Input: part model. Units: mm. Frame: model coordinates. A direction names the side the tool comes from. Give positions to 0.01 mm unless a question says otherwise; leave off trailing zeros. Loops run counter-clockwise (first coordinate to the right, second up) from the corner with the lowest first, then second, coordinate; pieces in that order, holes last. Notation, with made-up numbers: (26.5, 53) - (53.5, 53) arc R13 cw to (53.5, 72) - close; hole circle Ø11 at (-22.75, 12.25). An arc over 180 degrees is marked (long way). Answer as a JSON object with one key per item and string values.
from build123d import *

# Parameters (mm, degrees)
SKETCH1_W           = 106
SKETCH1_H           = 6
BOSS_EXTRUDE1_DEPTH = 6
SKETCH2_W           = 6
SKETCH2_H           = 20
SKETCH2_R           = 1.75
BOSS_EXTRUDE2_DEPTH = 6
FILLET1_R           = 2


with BuildPart() as part:
    # Sketch1 → Boss-Extrude1 (new body)
    with BuildSketch(Plane(origin=(0, 0, 0), x_dir=(1, 0, 0), z_dir=(0, 1, 0))):
        Rectangle(SKETCH1_W, SKETCH1_H)
    extrude(amount=BOSS_EXTRUDE1_DEPTH)

    # Sketch2 → Boss-Extrude2 (add)
    # profile 1 of 4: a face of its own
    with BuildSketch(Plane(origin=(0, 6, 0), x_dir=(1, 0, 0), z_dir=(0, 1, 0))):
        with Locations((-50, 13)):
            Rectangle(SKETCH2_W, SKETCH2_H)
        with Locations(Location((-50, 20, 0), (0, 0, 270))):
            Circle(SKETCH2_R, mode=Mode.SUBTRACT)
    # profile 2 of 4: a face of its own
    with BuildSketch(Plane(origin=(0, 6, 0), x_dir=(1, 0, 0), z_dir=(0, 1, 0))):
        with Locations((-50, -13)):
            Rectangle(SKETCH2_W, SKETCH2_H)
        with Locations(Location((-50, -20, 0), (0, 0, 90))):
            Circle(SKETCH2_R, mode=Mode.SUBTRACT)
    # profile 3 of 4: a face of its own
    with BuildSketch(Plane(origin=(0, 6, 0), x_dir=(1, 0, 0), z_dir=(0, 1, 0))):
        with Locations((50, -13)):
            Rectangle(SKETCH2_W, SKETCH2_H)
        with Locations(Location((50, -20, 0), (0, 0, 270))):
            Circle(SKETCH2_R, mode=Mode.SUBTRACT)
    # profile 4 of 4: a face of its own
    with BuildSketch(Plane(origin=(0, 6, 0), x_dir=(1, 0, 0), z_dir=(0, 1, 0))):
        with Locations((50, 13)):
            Rectangle(SKETCH2_W, SKETCH2_H)
        with Locations(Location((50, 20, 0), (0, 0, 90))):
            Circle(SKETCH2_R, mode=Mode.SUBTRACT)
    extrude(amount=-BOSS_EXTRUDE2_DEPTH)

    # Fillet1
    fillet1_edges = [part.edges().sort_by_distance(p)[0] for p in [
        (-47, 3, -3),
        (-47, 3, 3),
        (47, 3, 3),
        (47, 3, -3),
    ]]
    fillet(fillet1_edges, radius=FILLET1_R)


solid = part.part
Item 1: Cut plane B-B (x = 50). Return loops of the section in (y, z), then the cut area to 3 significant figures.
Geometry check:
{"outline": "(0, -23) - (6, -23) - (6, -21.75) - (0, -21.75) - close; (0, -18.25) - (6, -18.25) - (6, 18.25) - (0, 18.25) - close; (0, 21.75) - (6, 21.75) - (6, 23) - (0, 23) - close", "area": "234 mm2"}
Item 2: Cut plane C-C (y = 4.9). Return loops of the section in (x, z).
Geometry check:
{"outline": "(-53, -23) - (-47, -23) - (-47, -5) arc R2 cw to (-45, -3) - (45, -3) arc R2 cw to (47, -5) - (47, -23) - (53, -23) - (53, 23) - (47, 23) - (47, 5) arc R2 cw to (45, 3) - (-45, 3) arc R2 cw to (-47, 5) - (-47, 23) - (-53, 23) - close; hole circle Ø3.5 at (-50, -20); hole circle Ø3.5 at (-50, 20); hole circle Ø3.5 at (50, -20); hole circle Ø3.5 at (50, 20)"}
Item 3: Mould query, pull axis Z, two halves, no side actions, for faces 1 (the face through (51.71, 3.04, -19.62)), 2 (the face through (-50, 3, -23)), 3 (the face through (50, 3, 23)), 4 (the face through (47, 3, -14)). Classes: released by +Z, released by -Z, zero draft, split by the parting line, or undercut.
Geometry check:
{"face 1": "undercut", "face 2": "released by -Z", "face 3": "released by +Z", "face 4": "zero draft"}
Item 4: Material intervals for line 1 (X direction, y = 4.2, z = 20); line 2 (X direction, y = 2.8, z = -15.5); line 3 (Z direction, x = 33.5, y = 4.85), sorted ascending. Write a range as [from, to].
Geometry check:
{"line 1": "x = [-53, -51.75], [-48.25, -47], [47, 48.25], [51.75, 53]", "line 2": "x = [-53, -47], [47, 53]", "line 3": "z = [-3, 3]"}
Item 5: Cut plane D-D (z = -20). Return loops of the section in (x, y).
Geometry check:
{"outline": "(-53, 0) - (-51.75, 0) - (-51.75, 6) - (-53, 6) - close; (-48.25, 0) - (-47, 0) - (-47, 6) - (-48.25, 6) - close; (47, 0) - (48.25, 0) - (48.25, 6) - (47, 6) - close; (51.75, 0) - (53, 0) - (53, 6) - (51.75, 6) - close"}
Item 6: Cut plane A-A (z = 14.5). Return loops of the section in (x, y), then the cut area to 3 significant figures.
Geometry check:
{"outline": "(-53, 0) - (-47, 0) - (-47, 6) - (-53, 6) - close; (47, 0) - (53, 0) - (53, 6) - (47, 6) - close", "area": "72.0 mm2"}
Item 7: Contact query for flat-ended pins moving along their axis: P1, Ø2, axis at x = -1, y = 2.5, coming from the +Z side; P2, Ø2, axis at x = 50, z = 20, coming from the -Y side. Output: stop coordinate, or through.
Geometry check:
{"P1": "stops at z = 3", "P2": "passes through"}
Item 8: Access query for faces 5 (the face through (46.43, 2.96, 3.6)), 6 (the face through (-53, 3, 0)), 7 (the face through (-47, 3, -14)). Directions: +Z, -Z, +X, -X, +Y, -Y. A direction counts if a zero-diameter tool reaches every point of the face in a straight line with its end or side. Return the directions, or none.
Geometry check:
{"face 5": "+Z, +Y, -Y", "face 6": "+Z, -Z, -X, +Y, -Y", "face 7": "-Z, +Y, -Y"}
